Source: CAD feature listing. Evaluate the final solid. Frame: model axes, mm. Face numbers are marked on the shaded views. A direction names the side the tool comes from. Give positions to 0.01 mm unless a question says otherwise; leave off trailing zeros. Order: outer loops, then holes, each group sorted by start corner. A loop starts at its lowest first (then second) coordinate and runs counter-clockwise, first axis right, second up. Notation, with made-up numbers: (-14, 52.5) -> (35, 52.5) arc R22 ccw to (35, 80.5) -> close; hole circle Ø6 at (46.5, 65.5). An arc over 180 degrees is marked (long way). Use one line per item in the form item = value. Start each with the question number.
from build123d import *

# Parameters (mm, degrees)
SKETCH1_W           = 100
SKETCH1_H           = 40
BOSS_EXTRUDE1_DEPTH = 38
CUT_EXTRUDE2_START  = -12
SKETCH2_W           = 39.5
SKETCH2_H           = 34
CUT_EXTRUDE2_DEPTH  = 21
CUT_EXTRUDE3_DEPTH  = 9
CUT_EXTRUDE4_REACH  = 81.36
SKETCH4_R           = 2.4


with BuildPart() as part:
    # Sketch1 → Boss-Extrude1 (new body)
    with BuildSketch(Plane.XY):
        with Locations((16.25, 1.5625)):
            Rectangle(SKETCH1_W, SKETCH1_H)
    extrude(amount=BOSS_EXTRUDE1_DEPTH)

    # Sketch2 → Cut-Extrude2 (cut)
    with BuildSketch(Plane(origin=(0, 0, 0), x_dir=(-1, 0, 0), z_dir=(0, 0, -1)).offset(CUT_EXTRUDE2_START)):
        with Locations((-38.5, 1.5625)):
            Rectangle(SKETCH2_W, SKETCH2_H)
        with Locations((6, 1.5625)):
            Rectangle(SKETCH2_W, SKETCH2_H)
    extrude(amount=-CUT_EXTRUDE2_DEPTH, mode=Mode.SUBTRACT)

    # Sketch3 → Cut-Extrude3 (cut)
    with BuildSketch(Plane(origin=(-3.362318072, 0, 0), x_dir=(-1, 0, 0), z_dir=(0, 0, -1))):
        with BuildLine():
            ThreePointArc((-61.593370612, 1.614325749), (-20.676836723, -17.421621422), (21.715969185, -1.949710178))
            ThreePointArc((21.715969185, -1.949710178), (22.204299442, 9.465009595), (10.78957967, 9.953339852))
            ThreePointArc((10.78957967, 9.953339852), (-19.986233449, -1.278769909), (-49.690320582, 12.540715264))
            ThreePointArc((-49.690320582, 12.540715264), (-61.105040355, 13.029045522), (-61.593370612, 1.614325749))
        make_face()
    extrude(amount=-CUT_EXTRUDE3_DEPTH, mode=Mode.SUBTRACT)

    # Sketch4 → Cut-Extrude4 (cut, up to next)
    with BuildSketch(Plane(origin=(0, 0, 0), x_dir=(-1, 0, 0), z_dir=(0, 0, -1)), mode=Mode.PRIVATE) as cut_extrude4_sk1:
        with Locations((-62.25, 11.98479819)):
            Circle(SKETCH4_R)
    cut_extrude4_tool1 = extrude(cut_extrude4_sk1.sketch, amount=-CUT_EXTRUDE4_REACH, mode=Mode.PRIVATE) & part.part
    # Sketch4 → Cut-Extrude4 (cut, up to next)
    with BuildSketch(Plane(origin=(0, 0, 0), x_dir=(-1, 0, 0), z_dir=(0, 0, -1)), mode=Mode.PRIVATE) as cut_extrude4_sk2:
        with Locations((-62.25, -9.616561755)):
            Circle(SKETCH4_R)
    cut_extrude4_tool2 = extrude(cut_extrude4_sk2.sketch, amount=-CUT_EXTRUDE4_REACH, mode=Mode.PRIVATE) & part.part
    # Sketch4 → Cut-Extrude4 (cut, up to next)
    with BuildSketch(Plane(origin=(0, 0, 0), x_dir=(-1, 0, 0), z_dir=(0, 0, -1)), mode=Mode.PRIVATE) as cut_extrude4_sk3:
        with Locations((29.75, 11.98479819)):
            Circle(SKETCH4_R)
    cut_extrude4_tool3 = extrude(cut_extrude4_sk3.sketch, amount=-CUT_EXTRUDE4_REACH, mode=Mode.PRIVATE) & part.part
    # Sketch4 → Cut-Extrude4 (cut, up to next)
    with BuildSketch(Plane(origin=(0, 0, 0), x_dir=(-1, 0, 0), z_dir=(0, 0, -1)), mode=Mode.PRIVATE) as cut_extrude4_sk4:
        with Locations((29.75, -9.616561755)):
            Circle(SKETCH4_R)
    cut_extrude4_tool4 = extrude(cut_extrude4_sk4.sketch, amount=-CUT_EXTRUDE4_REACH, mode=Mode.PRIVATE) & part.part
    add(cut_extrude4_tool1.solids().sort_by_distance((62.25, 11.984798, 0))[0], mode=Mode.SUBTRACT)
    add(cut_extrude4_tool2.solids().sort_by_distance((62.25, -9.616562, 0))[0], mode=Mode.SUBTRACT)
    add(cut_extrude4_tool3.solids().sort_by_distance((-29.75, 11.984798, 0))[0], mode=Mode.SUBTRACT)
    add(cut_extrude4_tool4.solids().sort_by_distance((-29.75, -9.616562, 0))[0], mode=Mode.SUBTRACT)


solid = part.part
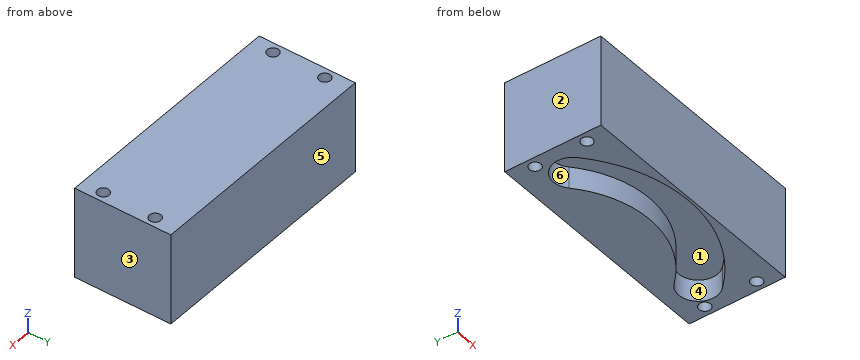
1) Cut plane D-D, the plane z = 28.5. Return the cut outline in (x, y), plus the area to 3 significant figures.
2) Pin query (flat end, axial travel): pin 1 (2 mm diameter, centred on x = 43.5, y = 3.5, fed in from -Z). Return the tip coordinate at first contact, or that it passes through.
3) Draft query along Y for the marked faces 3, 4, 5 and 6. Return one class per face: +Y half, -Y half, draft (parallel to the pull), parting line (faces both ways), or undercut.
4) Cut plane A-A, the plane x = -29.75. Return the cut outline in (y, z).
5) Cut plane C-C, the plane x = 24. Return the cut outline in (y, z).
6) Reachability of the marked faces 1 and 2 from +Z, -Z, +X, -X, +Y, -Y: full face, straight path, thin tool, end or side. Return the list, or none.
7) Material intervals for probe 1 along Y at (x, z) = (62.25, 24.5); probe 2 along X at (y, z) = (-5, 13); probe 3 along X at (y, z) = (12, 24.5), sorted ascending.
8) Cut plane B-B, the plane z = 10. Return the cut outline in (x, y).
Output values:
q1.outline = (-33.75, -18.44) -> (66.25, -18.44) -> (66.25, 21.56) -> (-33.75, 21.56) -> close; hole circle Ø4.8 at (-29.75, -9.62); hole circle Ø4.8 at (-29.75, 11.98); hole (-25.75, -15.44) -> (13.75, -15.44) -> (13.75, 18.56) -> (-25.75, 18.56) -> close; hole (18.75, -15.44) -> (58.25, -15.44) -> (58.25, 18.56) -> (18.75, 18.56) -> close; hole circle Ø4.8 at (62.25, -9.62); hole circle Ø4.8 at (62.25, 11.98)
q1.area = 1,240 mm^2
q2.pin_1 = 9
q3.face_3 = draft
q3.face_4 = undercut
q3.face_5 = +Y half
q3.face_6 = undercut
q4.outline = (-18.44, 0) -> (-12.02, 0) -> (-12.02, 38) -> (-18.44, 38) -> close; (-7.22, 0) -> (9.58, 0) -> (9.58, 38) -> (-7.22, 38) -> close; (14.38, 0) -> (21.56, 0) -> (21.56, 38) -> (14.38, 38) -> close
q5.outline = (-18.44, 0) -> (-16.75, 0) -> (-16.75, 9) -> (-0.32, 9) -> (-0.32, 0) -> (21.56, 0) -> (21.56, 38) -> (-18.44, 38) -> close; hole (-15.44, 12) -> (18.56, 12) -> (18.56, 33) -> (-15.44, 33) -> close
q6.face_1 = -Z
q6.face_2 = +Z, -Z, -X, +Y, -Y
q7.probe_1 = -18.44 to -12.02, -7.22 to 9.58, 14.38 to 21.56
q7.probe_2 = -33.75 to -25.75, 13.75 to 18.75, 58.25 to 66.25
q7.probe_3 = -33.75 to -32.15, -27.35 to -25.75, 13.75 to 18.75, 58.25 to 59.85, 64.65 to 66.25
q8.outline = (-33.75, -18.44) -> (66.25, -18.44) -> (66.25, 21.56) -> (-33.75, 21.56) -> close; hole circle Ø4.8 at (-29.75, -9.62); hole circle Ø4.8 at (-29.75, 11.98); hole circle Ø4.8 at (62.25, -9.62); hole circle Ø4.8 at (62.25, 11.98)
